```python
from build123d import *

# Parameters (mm, degrees)
F1_DEPTH = 800


with BuildPart() as f1:
    # F0 (on Right) → F1 (new body, symmetric)
    with BuildSketch(Plane.YZ):
        with BuildLine():
            Line((0, 120), (0, 0))
            Line((0, 0), (80, 0))
            Line((80, 0), (80, 4.5))
            ThreePointArc((80, 4.5), (78.389087, 8.389087), (74.5, 10))
            Line((74.5, 10), (21, 10))
            ThreePointArc((21, 10), (13.221825, 13.221825), (10, 21))
            Line((10, 21), (10, 114.5))
            ThreePointArc((10, 114.5), (8.389087, 118.389087), (4.5, 120))
            Line((4.5, 120), (0, 120))
        make_face()
    extrude(amount=F1_DEPTH, both=True)


solid = f1.part
```
Check sheet for the modelled part. Datum: model origin and axes. Units: mm. A direction names the side the tool comes from. Give positions to 0.01 mm unless a question says otherwise; leave off trailing zeros. Write each loop counter-clockwise with the first axis right and the second up, starting at its lowest first coordinate (ties: lowest second). Pieces come first, ordered by that corner, then holes. Notation, with made-up numbers: (73.5, 44.25) - (100.5, 44.25) arc R31 cw to (100.5, 79.25) - close; hole circle Ø5 at (46.25, 56). An arc over 180 degrees is marked (long way). Answer as a JSON object with one key per item and string values. Group by question number.
1) Sectioned sample at A-A (x = -636). Record the cut outline in (y, z), then the cut area to 3 significant figures.
2) Thickness scan on probe 1 along Y at (x, z) = (-307.5, 106); probe 2 along Y at (x, z) = (216.5, 17). Record the ranges inside material, lowest first. Write a range as from..to.
3) Access from +Z, -Z, +X, -X, +Y, -Y to the whole of each face (thin tool, end or side, straight path). Record for faces 1 (the face through (11, 10, 67)), 2 (the face through (11, 39, 0)).
4) Depth check by flat-ended pin: P1, Ø4, axis at x = -39.5, z = 47.5, coming from the +Y side; P2, Ø1, axis at x = -544, y = 28.5, coming from the +Z side. Enter the tip coordinate at first touch or a pass-through.
5) Sectioned sample at B-B (y = 59.5). Record the cut outline in (x, z).
Geometry results:
{
 "1": {"outline": "(0, 0) - (80, 0) - (80, 4.5) arc R5.5 ccw to (74.5, 10) - (21, 10) arc R11 cw to (10, 21) - (10, 114.5) arc R5.5 ccw to (4.5, 120) - (0, 120) - close", "area": "1,910 mm^2"},
 "2": {"probe 1": "y = 0..10", "probe 2": "y = 0..10.75"},
 "3": {"face 1": "+Z, +X, -X, +Y", "face 2": "-Z, +X, -X, +Y, -Y"},
 "4": {"P1": "stops at y = 10", "P2": "stops at z = 10"},
 "5": {"outline": "(-800, 0) - (800, 0) - (800, 10) - (-800, 10) - close"}
}
